from build123d import *

# Parameters (mm, degrees)
SKETCH1_W               = 60
SKETCH1_H               = 17.5
SKETCH3_R               = 15.75
CUT_EXTRUDE1_DEPTH      = 4
CUT_EXTRUDE2_DEPTH      = 25
CUT_EXTRUDE2_DEPTH_BACK = 25
SKETCH5_R               = 6
CUT_EXTRUDE3_DEPTH      = 65.903774929
SKETCH6_W               = 4
SKETCH6_H               = 4
CUT_EXTRUDE5_DEPTH      = 65.903774929


with BuildPart() as part:
    # Sketch1 → Revolve1 (revolve)
    with BuildSketch(Plane.XY, mode=Mode.PRIVATE) as revolve1_sk:
        with Locations((30, 8.75)):
            Rectangle(SKETCH1_W, SKETCH1_H)
    revolve(revolve1_sk.sketch.rotate(Axis((0, 0, 0), (-1, 0, 0)), 90), axis=Axis((0, 0, 0), (-1, 0, 0)))

    # Sketch3 → Cut-Extrude1 (cut)
    with BuildSketch(Plane(origin=(60, 0, 0), x_dir=(0, 0, -1), z_dir=(1, 0, 0))):
        Circle(SKETCH3_R)
    extrude(amount=-CUT_EXTRUDE1_DEPTH, mode=Mode.SUBTRACT)

    # Sketch4 → Cut-Extrude2 (cut, two sides: drawn at the far end of the back side and taken through both)
    with BuildSketch(Plane(origin=(56, 0, 0), x_dir=(0, 0, -1), z_dir=(1, 0, 0)).offset(-CUT_EXTRUDE2_DEPTH_BACK)):
        with BuildLine():
            Line((-8.45, 12.45), (8.45, 12.45))
            ThreePointArc((8.45, 12.45), (11.278427125, 11.278427125), (12.45, 8.45))
            Line((12.45, 8.45), (12.45, -8.45))
            ThreePointArc((12.45, -8.45), (11.278427125, -11.278427125), (8.45, -12.45))
            Line((8.45, -12.45), (-8.45, -12.45))
            ThreePointArc((-8.45, -12.45), (-11.278427125, -11.278427125), (-12.45, -8.45))
            Line((-12.45, -8.45), (-12.45, 8.45))
            ThreePointArc((-12.45, 8.45), (-11.278427125, 11.278427125), (-8.45, 12.45))
        make_face()
    extrude(amount=CUT_EXTRUDE2_DEPTH + CUT_EXTRUDE2_DEPTH_BACK, mode=Mode.SUBTRACT)

    # Sketch5 → Cut-Extrude3 (cut, through all)
    with BuildSketch(Plane.ZY):
        Circle(SKETCH5_R)
    extrude(amount=-CUT_EXTRUDE3_DEPTH, mode=Mode.SUBTRACT)

    # Sketch6 → Cut-Extrude5 (cut, through all)
    with BuildSketch(Plane.ZY):
        with Locations((0, 6)):
            Rectangle(SKETCH6_W, SKETCH6_H)
    extrude(amount=-CUT_EXTRUDE5_DEPTH, mode=Mode.SUBTRACT)


solid = part.part
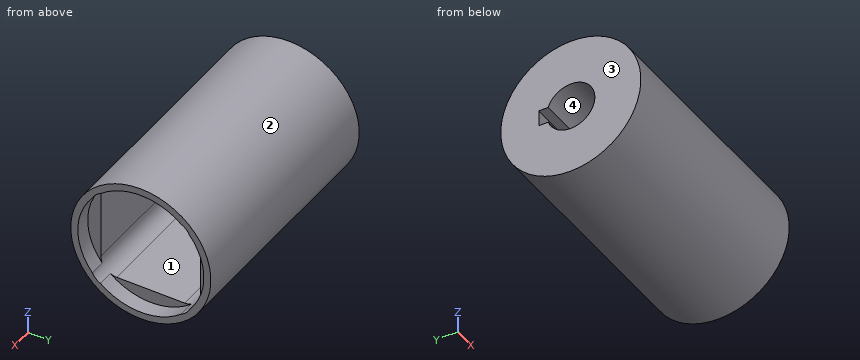
The model under review builds one solid part; all positions refer to its coordinate system, in mm. Face numbers are marked on the shaded views. Give positions to 0.01 mm unless a question says otherwise; leave off trailing zeros. Loops run counter-clockwise (first coordinate to the right, second up) from the corner with the lowest first, then second, coordinate; pieces in that order, holes last. Notation, with made-up numbers: (50.5, -22.5) -> (75.5, -22.5) arc R13 ccw to (75.5, 1.5) -> close; hole circle Ø4 at (47, 69.5). An arc over 180 degrees is marked (long way). Write each question's results on one line, items separated by ' | '.
1) Insertion check: pin 1 Ø1 at (y, z) = (-2, -8.5) entering from +X; pin 2 Ø4 at (y, z) = (-13, -2) entering from +X; pin 3 Ø1 at (x, z) = (34, -10) entering from +Y. Each pin has a flat end and moves straight along its axis. Give the tip position at first contact, or say it passes through.
Conclusion:
pin 1: stops at x = 31 | pin 2: stops at x = 56 | pin 3: stops at y = 14.7
2) Take a section at B-B, the plane z = -4. Give the boundary of the cut face in (x, y).
Conclusion:
outline: (0, -17.04) -> (60, -17.04) -> (60, -15.23) -> (56, -15.23) -> (56, -12.45) -> (31, -12.45) -> (31, -4.47) -> (0, -4.47) -> close; (0, 4.47) -> (31, 4.47) -> (31, 12.45) -> (56, 12.45) -> (56, 15.23) -> (60, 15.23) -> (60, 17.04) -> (0, 17.04) -> close
3) Take a section at D-D, the plane z = 14. Give the boundary of the cut face in (x, y).
Conclusion:
outline: (0, -10.5) -> (60, -10.5) -> (60, -7.22) -> (56, -7.22) -> (56, 7.22) -> (60, 7.22) -> (60, 10.5) -> (0, 10.5) -> close
4) Take a section at C-C, the plane x = 40. Give the boundary of the cut face in (y, z).
Conclusion:
outline: circle Ø35 at (0, 0); hole (-12.45, -8.45) arc R4 ccw to (-8.45, -12.45) -> (8.45, -12.45) arc R4 ccw to (12.45, -8.45) -> (12.45, 8.45) arc R4 ccw to (8.45, 12.45) -> (-8.45, 12.45) arc R4 ccw to (-12.45, 8.45) -> close
5) For line 1 along Y through (x, z) = (12, 0); line 2 along X through (y, z) = (-10, 9.5); line 3 along X through (y, z) = (6, 13.5), list the stretches that pass through material, from the lowest coordinate up. Write a range as from..to.
Conclusion:
line 1: y = -17.5..-6, 8..17.5 | line 2: x = 0..31 | line 3: x = 0..56
6) Take a section at A-A, the plane y = 0. Give the boundary of the cut face in (x, z).
Conclusion:
outline: (0, -17.5) -> (60, -17.5) -> (60, -15.75) -> (56, -15.75) -> (56, -12.45) -> (31, -12.45) -> (31, -6) -> (0, -6) -> close; (0, 6) -> (31, 6) -> (31, 12.45) -> (56, 12.45) -> (56, 15.75) -> (60, 15.75) -> (60, 17.5) -> (0, 17.5) -> close
7) Draft analysis for pull direction Z (two halves, no side actions). For the marked faces 1, 2, 3 and 4, state which applies: pulls with the +Z half, pulls with the -Z half, needs draft (parallel to the pull), parting line crosses it, or undercut.
Conclusion:
face 1: undercut | face 2: parting line crosses it | face 3: needs draft | face 4: undercut
